Build history of the part. All positions in model axes, mm. Face numbers are marked on the shaded views. A direction names the side the tool comes from. Give positions to 0.01 mm unless a question says otherwise; leave off trailing zeros. Order: outer loops, then holes, each group sorted by start corner. A loop starts at its lowest first (then second) coordinate and runs counter-clockwise, first axis right, second up. Notation, with made-up numbers: (24, 54) - (82, 54) arc R24 cw to (82, 77) - close; hole circle Ø6 at (62, -0.5). An arc over 180 degrees is marked (long way). Use a Markdown table: item, result.
from build123d import *

# Parameters (mm, degrees)
F0_R     = 4.95
F0_R_2   = 4.1
F1_DEPTH = 17
F2_DEPTH = 30
F3_SIZE  = 0.5


with BuildPart() as f1:
    # F0 (on Top) → F1 (new body)
    with BuildSketch(Plane.XY):
        Circle(F0_R)
        Circle(F0_R_2, mode=Mode.SUBTRACT)
        Circle(F0_R_2)
    extrude(amount=F1_DEPTH)

    # F0 (on Top) → F2 (join)
    with BuildSketch(Plane.XY):
        Circle(F0_R_2)
    extrude(amount=-F2_DEPTH)

    # F3
    f3_edges = [f1.edges().sort_by_distance(p)[0] for p in [
        (-4.95, 0, 17),
        (-4.1, 0, -30),
    ]]
    chamfer(f3_edges, length=F3_SIZE)


solid = f1.part
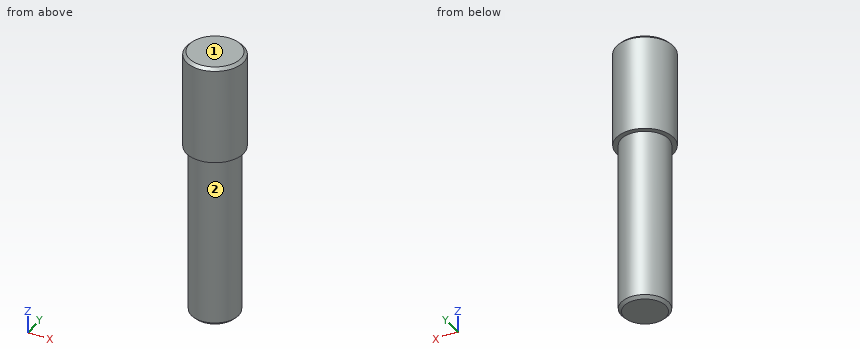
1) Wall check: line 1 (Y direction, x = 0, z = -3); line 2 (X direction, y = 1.5, z = 2); line 3 (X direction, y = -1.25, z = -24.5). Give the ranges that are in metal, low to high. Write a range as from..to.
Computed:
| item | result |
|---|---|
| line 1 | y = -4.1..4.1 |
| line 2 | x = -4.72..4.72 |
| line 3 | x = -3.9..3.9 |
2) Slice it at C-C (z = -8). Write the cut outline in (x, y).
Computed:
| item | result |
|---|---|
| outline | circle Ø8.2 at (0, 0) |
3) Slice it at A-A (x = 0). Write the cut outline in (y, z).
Computed:
| item | result |
|---|---|
| outline | (-4.95, 0) - (-4.1, 0) - (-4.1, -29.5) - (-3.6, -30) - (3.6, -30) - (4.1, -29.5) - (4.1, 0) - (4.95, 0) - (4.95, 16.5) - (4.45, 17) - (-4.45, 17) - (-4.95, 16.5) - close |
4) Tool access for the marked faces 1 and 2: list every direction of +Z, -Z, +X, -X, +Y, -Y with a clear straight run to the whole face (end or side of a thin tool).
Computed:
| item | result |
|---|---|
| face 1 | +Z, +X, -X, +Y, -Y |
| face 2 | -Z |
5) Pin check, flat tips, straight feed: P1, Ø4, axis at y = 3, z = -24, coming from the +X side; P2, Ø4, axis at x = -1, z = -15, coming from the +Y side; P3, Ø5, axis at y = 3, z = -14.5, coming from the -X side. Stop position of each tip, or through.
Computed:
| item | result |
|---|---|
| P1 | stops at x = 3.98 |
| P2 | stops at y = 4.1 |
| P3 | stops at x = -4.07 |
